```python
from build123d import *

# Parameters (mm, degrees)
EXTRUDE_1_DEPTH           = 20
SKETCH_2_R                = 4
CUT_EXTRUDE_1_DEPTH       = 52
FILLET_1_R                = 25
FILLET_2_R                = 5
FILLET_3_R                = 10
SKETCH_4_W                = 8
SKETCH_4_H                = 8
CUT_EXTRUDE_2_DEPTH       = 5
CUT_EXTRUDE_START         = -57
SKETCH_4_2_W              = 8
SKETCH_4_2_H              = 8
CUT_EXTRUDE_3_DEPTH       = 5
SKETCH_5_W                = 15
SKETCH_5_H                = 5
CUT_EXTRUDE_4_DEPTH       = 7.5
SKETCH_6_R                = 1.45
CUT_EXTRUDE_5_DEPTH       = 10
CUT_EXTRUDE_6_DEPTH       = 7
SKETCH_9_R                = 1.45
CUT_EXTRUDE_7_DEPTH       = 90
CUT_EXTRUDE_8_DEPTH       = 116.378724321
CUT_EXTRUDE_8_DEPTH_BACK  = 116.378724321
SKETCH_10_W               = 136.912738892
SKETCH_10_H               = 37.062753894
SKETCH_11_W               = 2.5
SKETCH_11_H               = 20
EXTRUDE_2_DEPTH           = 3
CUT_EXTRUDE_9_DEPTH       = 110.555003156
CUT_EXTRUDE_9_DEPTH_BACK  = 110.555003156
SKETCH_12_R               = 1.45
CUT_EXTRUDE_10_DEPTH      = 110.555003156
CUT_EXTRUDE_10_DEPTH_BACK = 1.5
CUT_EXTRUDE_10_START      = 3
SKETCH_13_R               = 3
CUT_EXTRUDE_11_DEPTH      = 1.5
CUT_EXTRUDE_11_DEPTH_BACK = 110.555003156
CUT_EXTRUDE_11_START      = -22
SKETCH_13_2_R             = 3
SKETCH_14_W               = 6
SKETCH_14_H               = 2
CUT_EXTRUDE_12_DEPTH      = 1.5


with BuildPart() as part:
    # Эскиз1 → Бобышка-Вытянуть1 (new body)
    with BuildSketch(Plane(origin=(0, 0, 0), x_dir=(1, 0, 0), z_dir=(0, 1, 0))):
        Polygon((21, 25), (-21, 25), (-21, 0), (-28.5, 0), (-28.5, 35), (-12.5, 62.5), (-12.5, 110), (12.5, 110), (12.5, 62.5), (28.5, 35), (28.5, 0), (21, 0), align=None)
    extrude(amount=EXTRUDE_1_DEPTH)

    # Эскиз2 → Вырез-Вытянуть1 (cut)
    with BuildSketch(Plane(origin=(28.5, 0, 0), x_dir=(0, 0, -1), z_dir=(1, 0, 0))):
        with Locations((10, 10)):
            Circle(SKETCH_2_R)
    extrude(amount=-CUT_EXTRUDE_1_DEPTH, mode=Mode.SUBTRACT)

    # Скругление1
    fillet_1_edges = [part.edges().sort_by_distance(p)[0] for p in [
        (28.5, 10, -35),
        (-28.5, 10, -35),
        (-12.5, 10, -62.5),
        (12.5, 10, -62.5),
    ]]
    fillet(fillet_1_edges, radius=FILLET_1_R)

    # Скругление2
    fillet_2_edges = [part.edges().sort_by_distance(p)[0] for p in [
        (28.5, 0, -14.128221453),
        (24.75, 0, 0),
        (-24.75, 0, 0),
        (-12.5, 0, -89.621778547),
        (-12.5, 20, -89.621778547),
        (28.5, 10, 0),
        (-28.5, 10, 0),
        (-24.75, 20, 0),
        (24.75, 20, 0),
        (-28.5, 0, -14.128221453),
        (-28.5, 20, -14.128221453),
        (20.5, 0, -48.75),
        (-20.5, 0, -48.75),
        (12.5, 0, -89.621778547),
        (27.637291802, 0, -34.76729112),
        (-27.637291802, 0, -34.76729112),
        (28.5, 20, -14.128221453),
        (-20.5, 20, -48.75),
        (20.5, 20, -48.75),
        (12.5, 20, -89.621778547),
        (27.637291802, 20, -34.76729112),
        (-27.637291802, 20, -34.76729112),
        (-13.362708198, 0, -62.73270888),
        (-13.362708198, 20, -62.73270888),
        (13.362708198, 0, -62.73270888),
        (13.362708198, 20, -62.73270888),
    ]]
    fillet(fillet_2_edges, radius=FILLET_2_R)

    # Скругление3
    fillet_3_edges = [part.edges().sort_by_distance(p)[0] for p in [
        (0, 0, -25),
        (0, 20, -25),
    ]]
    fillet(fillet_3_edges, radius=FILLET_3_R - 0.0001)  # a hair under: the kernel refuses the full size

    # Эскиз4 → Вырез-Вытянуть2 (cut)
    with BuildSketch(Plane(origin=(28.5, 0, 0), x_dir=(0, 0, -1), z_dir=(1, 0, 0))):
        with Locations((10, 10)):
            Rectangle(SKETCH_4_W, SKETCH_4_H)
    extrude(amount=-CUT_EXTRUDE_2_DEPTH, mode=Mode.SUBTRACT)

    # Эскиз4<2> → Вырез-Вытянуть3 (cut)
    with BuildSketch(Plane(origin=(28.5, 0, 0), x_dir=(0, 0, -1), z_dir=(1, 0, 0)).offset(CUT_EXTRUDE_START)):
        with Locations((10, 10)):
            Rectangle(SKETCH_4_2_W, SKETCH_4_2_H)
    extrude(amount=CUT_EXTRUDE_3_DEPTH, mode=Mode.SUBTRACT)

    # Эскиз5 → Вырез-Вытянуть4 (cut)
    with BuildSketch(Plane(origin=(0, 0, -110), x_dir=(-1, 0, 0), z_dir=(0, 0, -1))):
        with Locations((0, 17.5)):
            Rectangle(SKETCH_5_W, SKETCH_5_H)
        with Locations((0, 2.5)):
            Rectangle(SKETCH_5_W, SKETCH_5_H)
    extrude(amount=-CUT_EXTRUDE_4_DEPTH, mode=Mode.SUBTRACT)

    # Эскиз6 → Вырез-Вытянуть5 (cut)
    with BuildSketch(Plane(origin=(0, 15, 0), x_dir=(1, 0, 0), z_dir=(0, 1, 0))):
        with Locations(Location((-4, 106.25, 0), (0, 0, 270))):
            Circle(SKETCH_6_R)
        with Locations(Location((4, 106.25, 0), (0, 0, 90))):
            Circle(SKETCH_6_R)
    extrude(amount=-CUT_EXTRUDE_5_DEPTH, mode=Mode.SUBTRACT)

    # Эскиз8 → Вырез-Вытянуть6 (cut, symmetric)
    with BuildSketch(Plane(origin=(0, 0, 0), x_dir=(0, 0, -1), z_dir=(1, 0, 0))):
        with BuildLine():
            Line((102.5, 18), (37.5, 18))
            ThreePointArc((37.5, 18), (29.5, 10), (37.5, 2))
            Line((37.5, 2), (102.5, 2))
            Line((102.5, 2), (102.5, 18))
        make_face()
    extrude(amount=CUT_EXTRUDE_6_DEPTH, both=True, mode=Mode.SUBTRACT)

    # Эскиз9 → Вырез-Вытянуть7 (cut)
    with BuildSketch(Plane(origin=(0, 0, -110), x_dir=(-1, 0, 0), z_dir=(0, 0, -1))):
        with Locations((-10, 10)):
            Circle(SKETCH_9_R)
        with Locations((10, 10)):
            Circle(SKETCH_9_R)
    extrude(amount=-CUT_EXTRUDE_7_DEPTH, mode=Mode.SUBTRACT)

    # Эскиз10 → Вырез-Вытянуть8 (cut, two sides: drawn at the far end of the back side and taken through both)
    with BuildSketch(Plane(origin=(0, 0, 0), x_dir=(0, 0, -1), z_dir=(1, 0, 0)).offset(-CUT_EXTRUDE_8_DEPTH_BACK)):
        with Locations((61.52396192, 11.158211059)):
            Rectangle(SKETCH_10_W, SKETCH_10_H)
        with BuildLine():
            Line((37.5, 20), (102.5, 20))
            ThreePointArc((102.5, 20), (90.247548784, 16.26225608), (77.5, 15))
            Line((77.5, 15), (57.5, 15))
            ThreePointArc((57.5, 15), (47.192235936, 16.268943744), (37.5, 20))
        make_face(mode=Mode.SUBTRACT)
    extrude(amount=CUT_EXTRUDE_8_DEPTH + CUT_EXTRUDE_8_DEPTH_BACK, mode=Mode.SUBTRACT)

    # Эскиз11 → Бобышка-Вытянуть2 (add)
    with BuildSketch(Plane.XZ.offset(-15)):
        with Locations((8.25, -67.5)):
            Rectangle(SKETCH_11_W, SKETCH_11_H)
        with Locations((-8.25, -67.5)):
            Rectangle(SKETCH_11_W, SKETCH_11_H)
    extrude(amount=EXTRUDE_2_DEPTH)

    # Эскиз12 → Вырез-Вытянуть9 (cut, two sides: drawn at the far end of the back side and taken through both)
    with BuildSketch(Plane(origin=(9.5, 0, 0), x_dir=(0, 0, -1), z_dir=(1, 0, 0)).offset(-CUT_EXTRUDE_9_DEPTH_BACK)):
        with Locations(Location((67.5, 13.75, 0), (0, 0, 59.549685979))):
            Circle(SKETCH_12_R)
    extrude(amount=CUT_EXTRUDE_9_DEPTH + CUT_EXTRUDE_9_DEPTH_BACK, mode=Mode.SUBTRACT)

    # Эскиз13 → Вырез-Вытянуть10 (cut, two sides: drawn at the far end of the back side and taken through both)
    with BuildSketch(Plane(origin=(9.5, 0, 0), x_dir=(0, 0, -1), z_dir=(1, 0, 0)).offset(CUT_EXTRUDE_10_START - CUT_EXTRUDE_10_DEPTH_BACK)):
        with Locations((67.5, 13.75)):
            Circle(SKETCH_13_R)
    extrude(amount=CUT_EXTRUDE_10_DEPTH + CUT_EXTRUDE_10_DEPTH_BACK, mode=Mode.SUBTRACT)

    # Эскиз13<2> → Вырез-Вытянуть11 (cut, two sides: drawn at the far end of the back side and taken through both)
    with BuildSketch(Plane(origin=(9.5, 0, 0), x_dir=(0, 0, -1), z_dir=(1, 0, 0)).offset(CUT_EXTRUDE_11_START - CUT_EXTRUDE_11_DEPTH_BACK)):
        with Locations((67.5, 13.75)):
            Circle(SKETCH_13_2_R)
    extrude(amount=CUT_EXTRUDE_11_DEPTH + CUT_EXTRUDE_11_DEPTH_BACK, mode=Mode.SUBTRACT)

    # Эскиз14 → Вырез-Вытянуть12 (cut)
    with BuildSketch(Plane(origin=(0, 20, 0), x_dir=(1, 0, 0), z_dir=(0, 1, 0))):
        with Locations((0, 101.5)):
            Rectangle(SKETCH_14_W, SKETCH_14_H)
    extrude(amount=-CUT_EXTRUDE_12_DEPTH, mode=Mode.SUBTRACT)


solid = part.part
```
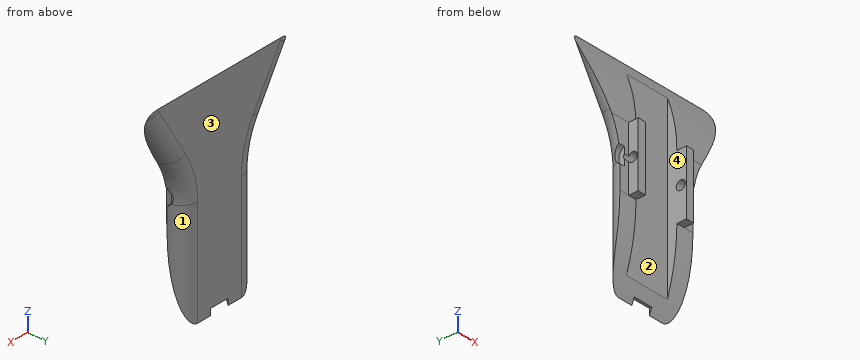
Can you work these out from the model? Positions are in its coordinate system, mm. Face numbers are marked on the shaded views. Coordinates: 2 decimals unless noted, no trailing zeros. Loops run counter-clockwise (first coordinate to the right, second up) from the corner with the lowest first, then second, coordinate; pieces in that order, holes last. Notation, with made-up numbers: (-18, 40.5) -> (3, 40.5) arc R29 ccw to (3, 74.5) -> close; hole circle Ø11 at (88.25, -8). An arc over 180 degrees is marked (long way). Put each result on its own line as item: value. Start each with the question number.
Q1. I want a section at B-B (z = -74.5). Write out the boundary of the cut face in (x, y), plus the area to 3 significant figures.
Q2. I want a section at D-D (z = -67.5). Count the separate pieces of the cut face and the enclosed holes in it, plus the area to 3 significant figures.
Q3. I'm going to push flat-ended pins straight in: P1, Ø2.5, axis at y = 13.75, z = -67.5, coming from the -X side; P2, Ø7, axis at x = 0.5, z = -60.5, coming from the -Y side; P3, Ø1, axis at y = 16, z = -70, coming from the -X side; P4, Ø1.8, axis at x = -13.5, z = -64.5, coming from the -Y side. Where does each tip first touch, or does it pass through?
Q4. Thinking about a two-plate mould opening in X: for the marked faces 1, 2, 3 and 4, which applies, pulls with the +X half, pulls with the -X half, needs draft (parallel to the pull), parting line crosses it, or undercut?
Q5. I want a section at C-C (x = -1.5). Write out the boundary of the cut face in (y, z).
Q6. If I drill on line 1 (Z direction, x = -8.35, y = 13.75); line 2 (Y direction, x = -7.85, z = -67.5); line 3 (X direction, y = 12.5, z = -71.5), over which ranges is the centre line in solid material (lowest first)? Write a range as [from, to].
Q7. I want a section at A-A (y = 13.75). Write out the boundary of the cut face in (x, z).
Taken from the geometry:
1. outline: (-12.5, 15) -> (-9.5, 15) -> (-9.5, 12) -> (-7, 12) -> (-7, 18) -> (7, 18) -> (7, 12) -> (9.5, 12) -> (9.5, 15) -> (12.5, 15) arc R5 ccw to (7.5, 20) -> (-7.5, 20) arc R5 ccw to start
1. area: 87.3 mm2
2. separate pieces: 3
2. enclosed holes: 0
2. area: 67.7 mm2
3. P1: passes through
3. P2: stops at y = 18
3. P3: stops at x = -12.47
3. P4: stops at y = 15
4. face 1: pulls with the +X half
4. face 2: undercut
4. face 3: needs draft
4. face 4: undercut
5. outline: (18, -97.02) arc R65 ccw to (19.21, -100.5) -> (20, -100.5) -> (20, -37.5) arc R42.5 ccw to (18, -41.82) -> close
6. line 1: z = [-77.5, -68.95], [-66.05, -57.5]
6. line 2: y = [12, 12.3], [15.2, 19.99]
6. line 3: x = [-9.5, -7], [7, 9.5]
7. outline: (-9.5, -77.5) -> (-7, -77.5) -> (-7, -68.95) -> (-9.5, -68.95) -> close; (-9.5, -66.05) -> (-7, -66.05) -> (-7, -57.5) -> (-9.5, -57.5) -> close; (7, -77.5) -> (9.5, -77.5) -> (9.5, -68.95) -> (7, -68.95) -> close; (7, -66.05) -> (9.5, -66.05) -> (9.5, -57.5) -> (7, -57.5) -> close
